The model under review builds one solid part; all positions refer to its coordinate system, in mm. A direction names the side the tool comes from. Give positions to 0.01 mm unless a question says otherwise; leave off trailing zeros. Order: outer loops, then holes, each group sorted by start corner. A loop starts at its lowest first (then second) coordinate and runs counter-clockwise, first axis right, second up. Notation, with made-up numbers: (60.25, 31.5) - (101.25, 31.5) arc R21 ccw to (101.25, 52.5) - close; hole circle Ø11 at (-20.75, 5). An arc over 180 degrees is marked (long way). Write item = value, one per line. Start each with the question number.
1. For P1, Ø1.5, axis at y = -4.5, z = 3, coming from the -X side; P2, Ø5, axis at x = 8, z = 6, coming from the +Y side; P3, Ø5, axis at y = -3, z = 18, coming from the -X side, all flat-tipped, find the tip position at first contact; note any pin that passes through.
2. We need section D-D, the plane x = 8. Give the boundary of the cut face in (y, z), and give its area (3 significant figures).
3. We need section C-C, the plane y = 0. Give the boundary of the cut face in (x, z), and give its area (3 significant figures).
4. Machinability: for faces 4 (the flat face through (4, -3, 0)), 5 (the flat face through (14.335, -3.48, 9.86)), 6 (the cylindrical face through (10.74, 2.9, 9.86)), 7 (the cylindrical face through (4.655, -2.222, 9.86)), 8 (the cylindrical face through (5.008, -3.159, 9.86)), which of the approach directions +Z, -Z, +X, -X, +Y, -Y give a long, thin tool a straight path to every point of the face, cutting with its end or side? Answer none if there is none.
5. Wall thickness on probe 1 along Y at (x, z) = (7.25, 10.5); probe 2 along Y at (x, z) = (0, 8); probe 3 along X at (y, z) = (-4, 3): over which ranges is each line inside the solid? List them lowest first.
6. We need section A-A, the plane x = 0. Give the boundary of the cut face in (y, z).
7. We need section B-B, the plane z = 10.5. Give the boundary of the cut face in (x, y), and give its area (3 significant figures).
8. Mouldability with a two-part tool opening along X and no side actions: class faces 1 (the cylindrical face through (10.84, 1.9, 9.86)), 2 (the cylindrical face through (10.302, -3.016, 9.86)), 3 (the flat face through (4, -3, 20)) as pulls with the +X half, pulls with the -X half, needs draft (parallel to the pull), parting line crosses it, or undercut.
from build123d import *

# Parameters (mm, degrees)
F1_DEPTH = 20


with BuildPart() as f1:
    # F0 (on Top) → F1 (new body)
    with BuildSketch(Plane.XY):
        with BuildLine():
            ThreePointArc((3.130612, -3.232533), (-4.498272, 0.124691), (3.304876, 3.054143))
            ThreePointArc((3.304876, 3.054143), (5.057214, 1.830866), (7.160258, 1.450997))
            ThreePointArc((7.160258, 1.450997), (10.896637, 1.91036), (14.5, 3))
            Line((14.5, 3), (14.129716, 3.928919))
            ThreePointArc((14.129716, 3.928919), (10.690142, 2.888807), (7.123599, 2.450325))
            ThreePointArc((7.123599, 2.450325), (5.441163, 2.75422), (4.039293, 3.732842))
            ThreePointArc((4.039293, 3.732842), (-5.497888, 0.1524), (3.826303, -3.950874))
            ThreePointArc((3.826303, -3.950874), (5.026855, -3.150465), (6.43329, -2.828101))
            ThreePointArc((6.43329, -2.828101), (10.356786, -3.023299), (14.175279, -3.94581))
            Line((14.175279, -3.94581), (14.5, -3))
            ThreePointArc((14.5, -3), (10.499674, -2.03356), (6.389346, -1.829067))
            ThreePointArc((6.389346, -1.829067), (4.631302, -2.232022), (3.130612, -3.232533))
        make_face()
    extrude(amount=F1_DEPTH)


solid = f1.part
Model answer:
q1.P1 = -4.02
q1.P2 = 2.85
q1.P3 = -5.48
q2.outline = (-2.82, 0) - (-1.82, 0) - (-1.82, 20) - (-2.82, 20) - close; (1.5, 0) - (2.5, 0) - (2.5, 20) - (1.5, 20) - close
q2.area = 40.1 mm2
q3.outline = (-5.5, 0) - (-4.5, 0) - (-4.5, 20) - (-5.5, 20) - close
q3.area = 20.0 mm2
q4.face_4 = -Z, +X, -X, +Y, -Y
q4.face_5 = +Z, -Z, +X, -Y
q4.face_6 = +Z, -Z, +Y
q4.face_7 = +Z, -Z
q4.face_8 = +Z, -Z, -Y
q5.probe_1 = -2.81 to -1.81, 1.45 to 2.46
q5.probe_2 = -5.5 to -4.5, 4.5 to 5.5
q5.probe_3 = -3.77 to -2.06, 2.06 to 3.77
q6.outline = (-5.5, 0) - (-4.5, 0) - (-4.5, 20) - (-5.5, 20) - close; (4.5, 0) - (5.5, 0) - (5.5, 20) - (4.5, 20) - close
q7.outline = (3.13, -3.23) arc R4.5 cw (long way) to (3.3, 3.05) arc R5 ccw to (7.16, 1.45) arc R22 ccw to (14.5, 3) - (14.13, 3.93) arc R21 cw to (7.12, 2.45) arc R4 cw to (4.04, 3.73) arc R5.5 ccw (long way) to (3.83, -3.95) arc R4 cw to (6.43, -2.83) arc R21 cw to (14.18, -3.95) - (14.5, -3) arc R22 ccw to (6.39, -1.83) arc R5 ccw to start
q7.area = 46.2 mm2
q8.face_1 = pulls with the +X half
q8.face_2 = undercut
q8.face_3 = needs draft
